Can you work these out from the model? Positions are in its coordinate system, mm. A direction names the side the tool comes from. Give positions to 0.01 mm unless a question says otherwise; leave off trailing zeros. Order: outer loops, then holes, each group sorted by start corner. A loop starts at its lowest first (then second) coordinate and runs counter-clockwise, first axis right, second up. Notation, with made-up numbers: M 4.5,41 L 23.5,41 A18 ccw 23.5,46 Z; hole C 79.25,-5 d1. An arc over 180 degrees is marked long. Write each question's results on one line, items separated by ' | '.
Autodesk Inventor part; units mm, degrees
ref_plane "YZ Plane" through (0, 0, 0) normal (1, 0, 0) x (0, 1, 0)
ref_plane "XZ Plane" through (0, 0, 0) normal (0, 1, 0) x (-1, 0, 0)
ref_plane "XY Plane" through (0, 0, 0) normal (0, 0, 1) x (1, 0, 0)
sketch "Sketch1" plane through (0, 0, 0) normal (0, 0, 1) x (1, 0, 0)
  circle A0 centre (0, 0) radius 2.5
  circle A1 centre (0, 0) radius 5
  line L0 (-30, 2.5) -> (30, 2.5)
  line L1 (-30, -2.5) -> (30, -2.5)
  line L2 (30, -2.5) -> (30, 2.5)
  line L3 (-30, 2.5) -> (-30, -2.5)
  dimension "d0" = 5
  dimension "d1" = 10
  dimension "d2" = 5
  dimension "d3" = 2.5
  dimension "d4" = 60
  dimension "d5" = 30
extrude "Extrusion1" add sketch "Sketch1" along normal blind 10 contours A0 L0 A1 L1 | A0 L1 A1 L0 | L0 A1 | L1 A1 | A1 L1 L3 L0 | L0 L2 L1 A1
sketch "Sketch2" plane through (4.3301, -2.5, 0) normal (0, -1, 0) x (1, 0, 0)
  line L0 (-8.6603, 10) -> (-8.6603, 0)
  line L1 (-34.3301, 10) -> (-8.6603, 10)
  line L2 (-34.3301, 0) -> (-34.3301, 10)
  line L3 (-8.6603, 0) -> (-34.3301, 0)
  line L4 (0, 0) -> (0, 10)
  line L5 (25.6699, 0) -> (0, 0)
  line L6 (25.6699, 0) -> (25.6699, 10)
  line L7 (0, 10) -> (25.6699, 10)
  circle A0 centre (-29.3301, 5) radius 2.5
  circle A1 centre (20.6699, 5) radius 2.5
  point P0 (-4.3301, 0)
  dimension "d8" = 5
  dimension "d9" = 5
  dimension "d10" = 5
  dimension "d11" = 5
  dimension "d12" = 5
  dimension "d13" = 5
extrude "Extrusion2" cut sketch "Sketch2" against normal blind 10 contours A0 | A1
properties part number "Y_Rail_Alignement _Connector_SquareBar-Rev3"
(1) Imagine slicing it at B-B, the plane x = 0. Write out the boundary of the cut face in (y, z), plus the area to 3 significant figures.
Data:
outline: M -5,0 L -2.5,0 L -2.5,10 L -5,10 Z; M 2.5,0 L 5,0 L 5,10 L 2.5,10 Z | area: 50.0 mm2
(2) For faces 4 (the face through (-17, 2.5, 5)), 5 (the face through (17, -2.5, 5)), 6 (the face through (17, 2.5, 5)), 7 (the face through (-17, -2.5, 5)), which set-ups out of +Z, -Z, +X, -X, +Y, -Y let a thin tool reach every point of the face, with its end or its side?
Data:
face 4: +Z, -Z, -X, +Y | face 5: +Z, -Z, +X, -Y | face 6: +Z, -Z, +X, +Y | face 7: +Z, -Z, -X, -Y
(3) I need wall thicknesses on L1, parallel to Z at x = -25, y = 1.2; L2, parallel to X at y = -0.25, z = 3; L3, parallel to Y at x = 26, z = 2.5. Which ranges of each line are inside material? Lowest first, please. Write a range as from..to.
Data:
L1: z = 0..2.5, 7.5..10 | L2: x = -30..-26.5, -23.5..-2.49, 2.49..23.5, 26.5..30 | L3: y = -2.5..2.5
(4) Imagine slicing it at D-D, the plane x = 23. Write out the boundary of the cut face in (y, z), plus the area to 3 significant figures.
Data:
outline: M -2.5,0 L 2.5,0 L 2.5,3.5 L -2.5,3.5 Z; M -2.5,6.5 L 2.5,6.5 L 2.5,10 L -2.5,10 Z | area: 35.0 mm2
(5) Imagine slicing it at C-C, the plane z = 1.75. Write out the boundary of the cut face in (x, y), plus the area to 3 significant figures.
Data:
outline: M -30,-2.5 L -4.33,-2.5 A5 ccw 4.33,-2.5 L 30,-2.5 L 30,2.5 L 4.33,2.5 A5 ccw -4.33,2.5 L -30,2.5 Z; hole C 0,0 d5 | area: 311 mm2
(6) We'd pull the mould along Z, two halves only. Please class faces 1 (the face through (0, -5, 5)), 2 (the face through (0, 3, 10)), 3 (the face through (23.16, -0.04, 6.69)): +Z half, -Z half, draft (parallel to the pull), parting line (faces both ways), or undercut.
Data:
face 1: draft | face 2: +Z half | face 3: undercut
(7) Imagine slicing it at A-A, the plane y = 0. Write out the boundary of the cut face in (x, z).
Data:
outline: M -30,0 L -2.5,0 L -2.5,10 L -30,10 Z; M 2.5,0 L 30,0 L 30,10 L 2.5,10 Z; hole C -25,5 d5; hole C 25,5 d5
(8) Will these pins go through, and if not, where does the flat tip stop? P1, Ø3, axis at x = -20, z = 3.5, coming from the -Y side; P2, Ø5, axis at x = -14, z = 5.5, coming from the +Y side; P3, Ø3, axis at x = 3, z = 6, coming from the +Y side.
Data:
P1: stops at y = -2.5 | P2: stops at y = 2.5 | P3: stops at y = 4.77
